For this review, take the finished solid that the model builds, in its own axes (mm). Face numbers are marked on the shaded views. A direction names the side the tool comes from. Coordinates: 2 decimals unless noted, no trailing zeros. Write each loop counter-clockwise with the first axis right and the second up, starting at its lowest first coordinate (ties: lowest second). Pieces come first, ordered by that corner, then holes.
```python
from build123d import *

# Parameters (mm, degrees)
SKETCH_W     = 40
SKETCH_H     = 10
PAD_DEPTH    = 2
PAD001_DEPTH = 5
SKETCH002_W  = 2
SKETCH002_H  = 6
PAD002_DEPTH = 1


with BuildPart() as part:
    # Sketch → Pad (new body)
    with BuildSketch(Plane.XY):
        with Locations((20, 5)):
            Rectangle(SKETCH_W, SKETCH_H)
    extrude(amount=PAD_DEPTH)

    # Sketch001 → Pad001 (new body)
    with BuildSketch(Plane.XY.offset(2)):
        Polygon((18.5, 2.1), (18.5, 5), (18.5, 7.9), (21.5, 7.9), (21.5, 2.1), (20, 2.1), align=None)
    extrude(amount=PAD001_DEPTH)

    # Sketch002 → Pad002 (new body)
    with BuildSketch(Plane.XY.offset(2)):
        with Locations((3, 5)):
            Rectangle(SKETCH002_W, SKETCH002_H)
        with Locations((8.5, 5)):
            Rectangle(SKETCH002_W, SKETCH002_H)
        with Locations((14, 5)):
            Rectangle(SKETCH002_W, SKETCH002_H)
        with Locations((26, 5)):
            Rectangle(SKETCH002_W, SKETCH002_H)
        with Locations((31.5, 5)):
            Rectangle(SKETCH002_W, SKETCH002_H)
        with Locations((37, 5)):
            Rectangle(SKETCH002_W, SKETCH002_H)
    extrude(amount=PAD002_DEPTH)


solid = part.part
```
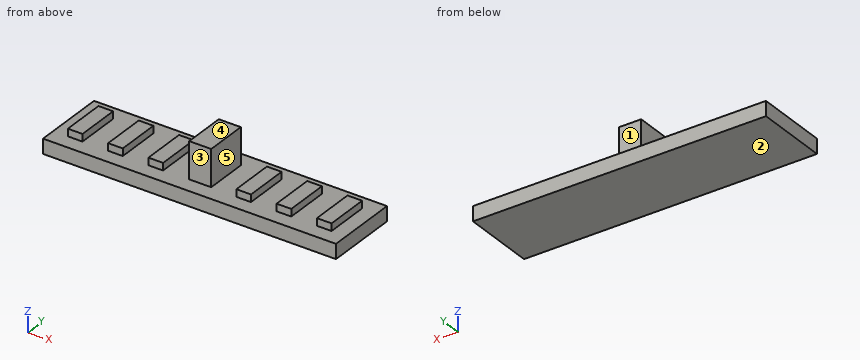
1) Consider section B-B (x = 20.5). Give the boundary of the cut face in (y, z).
2) Consider section C-C (z = 4.75). Give the boundary of the cut face in (x, y).
3) For L1, parallel to Z at x = 30, y = 4.5; L2, parallel to X at y = 2.25, z = 6.5; L3, parallel to Z at x = 14, y = 3, list the stretches that pass through material, from the lowest coordinate up.
4) Tool access review of the marked faces 1, 2, 3, 4 and 5: name each direction out of +Z, -Z, +X, -X, +Y, -Y from which nothing blocks a thin tool from reaching the whole face with its end or side.
5) Clearance check with flat-ended pins moving along their axes: P1, Ø1, axis at x = 31.5, y = 6.5, coming from the +Z side; P2, Ø0.5, axis at x = 14, z = 2.5, coming from the -Y side; P3, Ø1.5, axis at x = 12, y = 4, coming from the +Z side. State where each tip first meets the part, or that it passes through.
6) Consider section D-D (y = 1.5). Give the boundary of the cut face in (x, z).
Results:
1. outline: (0, 0) - (10, 0) - (10, 2) - (7.9, 2) - (7.9, 7) - (2.1, 7) - (2.1, 2) - (0, 2) - close
2. outline: (18.5, 2.1) - (21.5, 2.1) - (21.5, 7.9) - (18.5, 7.9) - close
3. L1: z = 0 to 2
3. L2: x = 18.5 to 21.5
3. L3: z = 0 to 3
4. face 1: +Z, +Y
4. face 2: -Z, +X, -X, +Y, -Y
4. face 3: +Z, -Y
4. face 4: +Z, +X, -X, +Y, -Y
4. face 5: +Z, +Y, -Y
5. P1: stops at z = 3
5. P2: stops at y = 2
5. P3: stops at z = 2
6. outline: (0, 0) - (40, 0) - (40, 2) - (0, 2) - close
